Autodesk Inventor part; units mm, degrees
ref_plane "Work Plane1" through (-65.75, 0, 74) normal (0, 0, 1) x (1, 0, 0)
ref_plane "YZ Plane" through (0, 0, 0) normal (1, 0, 0) x (0, 1, 0)
ref_plane "XZ Plane" through (0, 0, 0) normal (0, 1, 0) x (-1, 0, 0)
sketch "Sketch1" plane through (0, 0, 0) normal (0, 1, 0) x (-1, 0, 0)
  circle A0 centre (0, 0) radius 2.6
  circle A1 centre (-20, 0) radius 2.6
  circle A2 centre (0, 148) radius 2.6
  circle A3 centre (-20, 148) radius 2.6
  circle A4 centre (29.75, -4) radius 2.6
  line L0 (29.75, -4) -> (29.75, -1.4) construction
  line L1 (29.75, -4) -> (32.35, -4) construction
  circle A5 centre (29.75, 28) radius 2.6
  circle A6 centre (65.75, -4) radius 2.6
  circle A7 centre (65.75, 28) radius 2.6
  line L2 (0, 74) -> (-20, 74) construction
  circle A8 centre (26, 54) radius 2.6
  circle A9 centre (42, 54) radius 2.6
  circle A10 centre (26, 94) radius 2.6
  circle A11 centre (42, 94) radius 2.6
  circle A12 centre (29.75, 152) radius 2.6
  circle A13 centre (29.75, 120) radius 2.6
  circle A14 centre (65.75, 152) radius 2.6
  circle A15 centre (65.75, 120) radius 2.6
  circle A16 centre (65.75, -4) radius 7.3625 construction
  circle A17 centre (65.75, 152) radius 7.3625 construction
  circle A18 centre (29.75, 152) radius 7.3625 construction
  circle A19 centre (-20, 148) radius 7.3625 construction
  circle A20 centre (-20, 0) radius 7.3625 construction
  circle A21 centre (29.75, -4) radius 7.3625 construction
  line L3 (73.1125, 152) -> (73.1125, -4)
  line L4 (65.75, -11.3625) -> (29.75, -11.3625)
  line L5 (-20.5901, -7.3388) -> (29.1599, -11.3388)
  line L6 (65.75, 159.3625) -> (29.75, 159.3625)
  line L7 (29.1599, 159.3388) -> (-20.5901, 155.3388)
  line L8 (-27.3625, 148) -> (-27.3625, 0)
  arc A22 (65.75, -11.3625) -> (73.1125, -4) centre (65.75, -4) ccw
  arc A23 (73.1125, 152) -> (65.75, 159.3625) centre (65.75, 152) ccw
  arc A24 (29.75, 159.3625) -> (29.1599, 159.3388) centre (29.75, 152) ccw
  arc A25 (-27.3625, 0) -> (-20.5901, -7.3388) centre (-20, 0) ccw
  arc A26 (-20.5901, 155.3388) -> (-27.3625, 148) centre (-20, 148) ccw
  arc A27 (29.1599, -11.3388) -> (29.75, -11.3625) centre (29.75, -4) ccw
  point P0 (29.75, 30.6)
  point P1 (32.35, 28)
  point P2 (65.75, -1.4)
  point P3 (68.35, -4)
  point P4 (65.75, 30.6)
  point P5 (68.35, 28)
  dimension "d0" = 5.2
  dimension "d1" = 20
  dimension "d2" = 148
  dimension "d3" = 4
  dimension "d4" = 29.75
  dimension "d7" = 32
  dimension "d10" = 36
  dimension "d13" = 74
  dimension "d18" = 16
  dimension "d21" = 40
  dimension "d24" = 20
  dimension "d25" = 26
  dimension "d26" = 4.7625
extrude "Extrusion1" add sketch "Sketch1" along normal blind 4.7625
ref_plane "Work Plane1" through (-65.75, 0, 74) normal (0, 0, 1) x (1, 0, 0)
sketch "Sketch3" plane through (0, 4.7625, 0) normal (0, 1, 0) x (1, 0, 0)
  arc A0 (-29.75, -159.3625) -> (-29.1599, -159.3388) centre (-29.75, -152) ccw
  line L0 (-29.1599, -159.3388) -> (20.5901, -155.3388)
  arc A1 (20.5901, -155.3388) -> (27.3625, -148) centre (20, -148) ccw
  line L1 (27.3625, -148) -> (27.3625, 0)
  arc A2 (27.3625, 0) -> (20.5901, 7.3388) centre (20, 0) ccw
  line L2 (20.5901, 7.3388) -> (-29.1599, 11.3388)
  arc A3 (-29.1599, 11.3388) -> (-29.75, 11.3625) centre (-29.75, 4) ccw
  line L3 (-29.75, 11.3625) -> (-65.75, 11.3625)
  arc A4 (-65.75, 11.3625) -> (-73.1125, 4) centre (-65.75, 4) ccw
  line L4 (-73.1125, 4) -> (-73.1125, -152)
  arc A5 (-73.1125, -152) -> (-65.75, -159.3625) centre (-65.75, -152) ccw
  line L5 (-65.75, -159.3625) -> (-29.75, -159.3625)
  circle A6 centre (-29.75, -152) radius 2.6
  circle A7 centre (-65.75, -120) radius 2.6
  circle A8 centre (-26, -94) radius 2.6
  circle A9 centre (-42, -54) radius 2.6
  circle A10 centre (-26, -54) radius 2.6
  circle A11 centre (-65.75, -28) radius 2.6
  circle A12 centre (-29.75, -28) radius 2.6
  circle A13 centre (-29.75, 4) radius 2.6
  circle A14 centre (0, -148) radius 2.6
  circle A15 centre (0, 0) radius 2.6
  circle A16 centre (-42, -94) radius 2.6
  circle A17 centre (-29.75, -120) radius 2.6
  circle A18 centre (-65.75, -152) radius 2.6
  circle A19 centre (-65.75, 4) radius 2.6
  circle A20 centre (20, -148) radius 2.6
  circle A21 centre (20, 0) radius 2.6
  circle A22 centre (0, -113) radius 2.6
  circle A23 centre (20, -113) radius 2.6
  circle A24 centre (0, 0) radius 2.6
  line L6 (-73.1125, -74) -> (27.3625, -74) construction
  line L7 (27.3625, -148) -> (27.3625, 0) construction
  circle A25 centre (0, -35) radius 2.6
  circle A26 centre (20, -35) radius 2.6
  dimension "d56" = 148
  dimension "d60" = 35
  dimension "d61" = 74
extrude "Extrusion3" cut sketch "Sketch3" against normal through all contours A22 | A23
extrude "Extrusion4" cut sketch "Sketch3" against normal through all contours A25 | A26
equation "\"d13\" = 0.5 * d2"
equation "\"d24\" = 0.5 * d21"
properties part number "CNC-014-ZAxisSubMount1" material "Aluminum 5052"
Design review of the part built by this model. Coordinates are the model's own, in mm. Round coordinates to 2 decimals unless told otherwise and drop trailing zeros. Write each loop counter-clockwise with the first axis right and the second up, starting at its lowest first coordinate (ties: lowest second). Pieces come first, ordered by that corner, then holes. Notation, with made-up numbers: (-18.75, 28) -> (1.25, 28) arc R22 ccw to (1.25, 39) -> close; hole circle Ø1 at (-18.5, 19). An arc over 180 degrees is marked (long way). One line per question, with ' | ' between items.
(1) Insertion check: P1, Ø6, axis at x = 20, z = 113, coming from the +Y side. The pin has a flat end and moves straight along its axis. Give the tip position at first contact, or say it passes through.
Result sheet:
P1: y = 4.76
(2) Take a section at B-B, the plane x = 10.5. State the section outline as (y, z) points, and give its area (3 significant figures).
Result sheet:
outline: (0, -8.15) -> (4.76, -8.15) -> (4.76, 156.15) -> (0, 156.15) -> close | area: 782 mm2
(3) Draft analysis for pull direction Z (two halves, no side actions). For faces 1 (the cylindrical face through (-27.153, 2.348, 27.886)), 2 (the flat face through (-48, 2, -11.362)), 3 (the flat face through (-22, 4.762, 75)), state which applies: released by +Z, released by -Z, zero draft, split by the parting line, or undercut.
Result sheet:
face 1: undercut | face 2: released by -Z | face 3: zero draft
(4) Take a section at A-A, the plane y = 2.9. State how many separate pieces and enclosed holes the cut face has, and give its area (3 significant figures).
Result sheet:
separate pieces: 1 | enclosed holes: 20 | area: 16,400 mm2
(5) Wall thickness on line 1 (Z direction, x = -42, y = 3.1); line 2 (Z direction, x = -29.75, y = 1.9); line 3 (X direction, y = 3.5, z = 113): over which ranges is each line inside the solid? List them lowest first. Write a range as [from, to].
Result sheet:
line 1: [-11.36, 51.4], [56.6, 91.4], [96.6, 159.36] | line 2: [-11.36, -6.6], [-1.4, 25.4], [30.6, 117.4], [122.6, 149.4], [154.6, 159.36] | line 3: [-73.11, -2.6], [2.6, 17.4], [22.6, 27.36]
